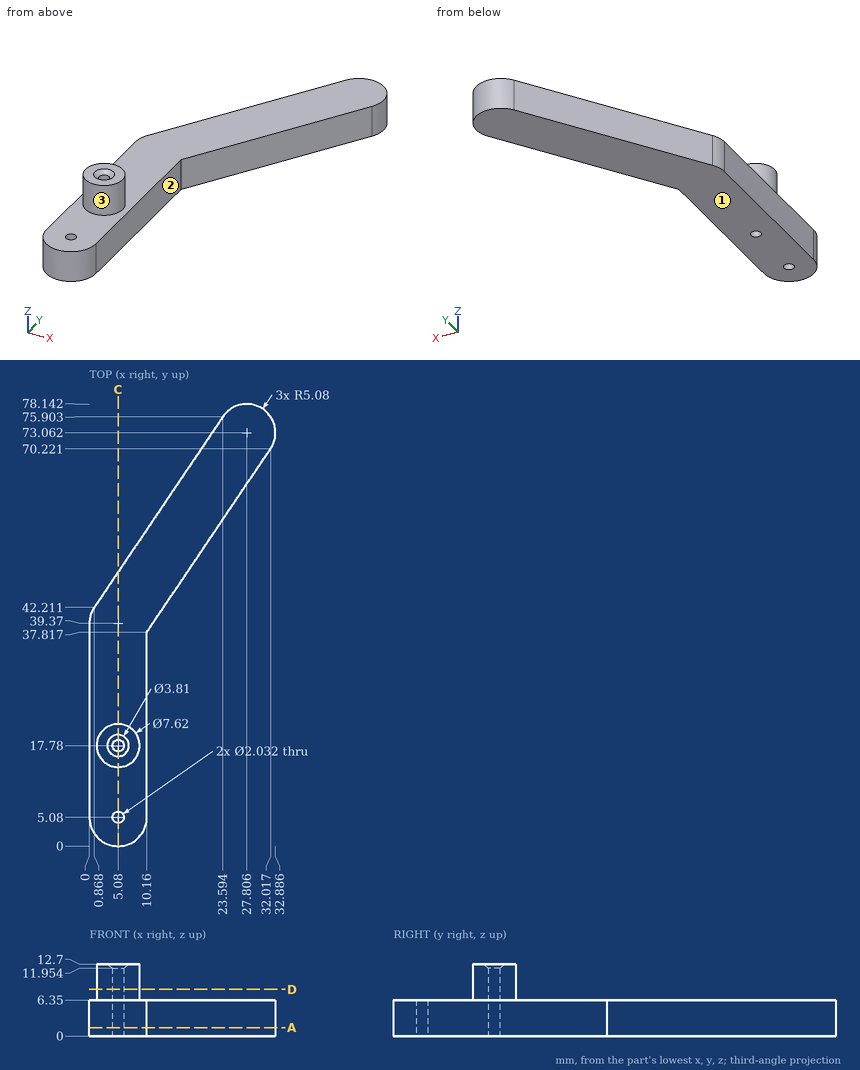
Drawing for the job (mm, zero at the part's lowest x, y, z). A direction names the side the tool comes from. Give positions to 0.01 mm unless a question says otherwise; leave off trailing zeros. Order: outer loops, then holes, each group sorted by start corner. A loop starts at its lowest first (then second) coordinate and runs counter-clockwise, first axis right, second up. Notation, with made-up numbers: M 12,78.5 L 23,78.5 A24 ccw 23,94.5 Z; hole C 27.5,-40 d2. An arc over 180 degrees is marked long. Put each result on its own line as item: value.
Item 1: 3-axis set-ups, long thin cutter, end or side, ignore diameter. For the marked faces 1, 2 and 3: which of +Z, -Z, +X, -X, +Y, -Y reach the whole face in a straight line?
From the geometry:
face 1: -Z, +X, -X, +Y, -Y
face 2: +Z, -Z, +X, -Y
face 3: +Z
Item 2: Slice it at C-C, the plane x = 5.08. Give the number of separate pieces and of enclosed holes in the cut face, plus the area to 3 significant figures.
From the geometry:
separate pieces: 3
enclosed holes: 0
area: 317 mm2
Item 3: Slice it at D-D, the plane z = 8.25. Write the cut outline in (x, y).
From the geometry:
outline: C 5.08,17.78 d7.62; hole C 5.08,17.78 d2.03
Item 4: Flat gauge pins, fed straight in: pin 1 Ø6 at (x, z) = (18, 8.5) entering from -Y (1 decimal); pin 2 Ø7 at (y, z) = (15, 2) entering from +X; pin 3 Ø1 at (y, z) = (68, 2) entering from -X (1 decimal). Where does each tip first touch, or does it go through?
From the geometry:
pin 1: stops at y = 46.3
pin 2: stops at x = 10.16
pin 3: stops at x = 17.9
Item 5: Probe line 1 (X direction, y = 17.78, z = 5.75) (1 decimal); line 2 (Y direction, x = 5.08, z = 2.5) (1 decimal); line 3 (Y direction, x = 5.08, z = 8.75) (1 decimal). List the from-to ranges inside material, lowest first. Write a range as [from, to].
From the geometry:
line 1: x = [0, 4.1], [6.1, 10.2]
line 2: y = [0, 4.1], [6.1, 16.8], [18.8, 48.5]
line 3: y = [14, 16.8], [18.8, 21.6]
Item 6: Slice it at A-A, the plane z = 1.5. Write the cut outline in (x, y) (1 decimal).
From the geometry:
outline: M 0,5.1 A5.1 ccw 10.2,5.1 L 10.2,37.8 L 32,70.2 A5.1 ccw 23.6,75.9 L 0.9,42.2 A5.1 ccw 0,39.4 Z; hole C 5.1,5.1 d2; hole C 5.1,17.8 d2
